Could you check a few things on this model? Use its own coordinates, in mm. A direction names the side the tool comes from. Coordinates: 2 decimals unless noted, no trailing zeros. Order: outer loops, then holes, each group sorted by start corner. A loop starts at its lowest first (then second) coordinate and runs counter-clockwise, first axis right, second up. Notation, with made-up numbers: M 6,-22.75 L 46,-22.75 A15 ccw 46,-3.75 Z; hole C 59,71.5 d8. An arc over 180 degrees is marked long. Put each result on its own line as item: value. Start each with the question number.
```python
from build123d import *

# Parameters (mm, degrees)
SKETCH_1_W               = 370
SKETCH_1_H               = 370
EXTRUDE_1_DEPTH          = 15
SKETCH_2_W               = 155
SKETCH_2_H               = 155
CUT_EXTRUDE_1_DEPTH      = 20
HOLE_WIZARD_1_AT_2_COUNT = 2
HOLE_WIZARD_1_AT_2_PITCH = 320
HOLE_WIZARD_1_AT_3_COUNT = 2
HOLE_WIZARD_1_AT_3_PITCH = 226.27416998
HOLE_WIZARD_1_AT_4_COUNT = 2
HOLE_WIZARD_1_AT_4_PITCH = 226.27416998
MM_1_D                   = 20
MM_1_DEPTH               = 17
MM_1_CSINK_D             = 20.05
MM_1_CSINK_ANGLE         = 90
MM_1_TIP                 = 6.00860619


with BuildPart() as part:
    # 草图1 → 凸台-拉伸1 (new body)
    with BuildSketch(Plane.XY):
        Rectangle(SKETCH_1_W, SKETCH_1_H)
    extrude(amount=EXTRUDE_1_DEPTH)

    # 草图2 → 切除-拉伸1 (cut)
    with BuildSketch(Plane.XY.offset(15)):
        with Locations((107.5, 107.5)):
            Rectangle(SKETCH_2_W, SKETCH_2_H)
        with Locations((-107.5, 107.5)):
            Rectangle(SKETCH_2_W, SKETCH_2_H)
        with Locations((-107.5, -107.5)):
            Rectangle(SKETCH_2_W, SKETCH_2_H)
        with Locations((107.5, -107.5)):
            Rectangle(SKETCH_2_W, SKETCH_2_H)
    extrude(amount=-CUT_EXTRUDE_1_DEPTH, mode=Mode.SUBTRACT)

    # 草图4 → 打孔尺寸(%根据)内六角圆柱头螺钉的类型1 (revolve, cut)
    with BuildSketch(Plane(origin=(-160, 0, 15), x_dir=(0, -1, 0), z_dir=(1, 0, 0))):
        Polygon((0, 0), (0, 20.304733405), (5.5, 17), (5.5, 11), (9, 11), (9, 0.025), (9.025, 0), align=None)
    hole_wizard_1 = revolve(axis=Axis((-160, 0, 21.35), (0, 0, -1)), mode=Mode.SUBTRACT)

    # 打孔尺寸(%根据)内六角圆柱头螺钉的类型1 at 2: 打孔尺寸(%根据)内六角圆柱头螺钉的类型1 ×2
    with Locations(*[(i * HOLE_WIZARD_1_AT_2_PITCH, 0, 0) for i in range(1, HOLE_WIZARD_1_AT_2_COUNT)]):
        add(hole_wizard_1, mode=Mode.SUBTRACT)

    # 打孔尺寸(%根据)内六角圆柱头螺钉的类型1 at 3: 打孔尺寸(%根据)内六角圆柱头螺钉的类型1 ×2
    with Locations(*[Vector(0.707106781, 0.707106781, 0) * (i * HOLE_WIZARD_1_AT_3_PITCH) for i in range(1, HOLE_WIZARD_1_AT_3_COUNT)]):
        add(hole_wizard_1, mode=Mode.SUBTRACT)

    # 打孔尺寸(%根据)内六角圆柱头螺钉的类型1 at 4: 打孔尺寸(%根据)内六角圆柱头螺钉的类型1 ×2
    with Locations(*[Vector(0.707106781, -0.707106781, 0) * (i * HOLE_WIZARD_1_AT_4_PITCH) for i in range(1, HOLE_WIZARD_1_AT_4_COUNT)]):
        add(hole_wizard_1, mode=Mode.SUBTRACT)

    # 大小mm 暗销槽口1
    with Locations(Plane.XY.offset(15)):
        with Locations((0, 0)):
            CounterSinkHole(MM_1_D / 2, MM_1_CSINK_D / 2, depth=MM_1_DEPTH, counter_sink_angle=MM_1_CSINK_ANGLE)
            with Locations((0, 0, -(MM_1_DEPTH + MM_1_TIP / 2))):  # 118° drill point
                Cone(0, MM_1_D / 2, MM_1_TIP, mode=Mode.SUBTRACT)


solid = part.part
```
Item 1: I need wall thicknesses on probe 1 along X at (y, z) = (0, 3.15); probe 2 along X at (y, z) = (0, 9). Which ranges of each line are inside material? Lowest first, please.
Item 2: For pin 1 Ø20 at (x, y) = (1.5, -163) entering from +Z; pin 2 Ø4.5 at (y, z) = (-101.5, 9) entering from -X; pin 3 Ø7.5 at (x, z) = (77.5, 4.5) entering from +Y; pin 4 Ø4.5 at (x, z) = (-74, 7.5) entering from -Y, each with a flat end and sliding along its axis, tell me the tip position at first contact or that it passes through.
Item 3: If we mould it in two halves opening along Y, with no side actions, what happens to faces 4 (the flat face through (0, 185, 7)), 5 (the flat face through (-185, 0, 7)), 6 (the cylindrical face through (-154.63, 1.19, 2.03))? For each: released by +Y, released by -Y, zero draft, split by the parting line, or undercut.
Item 4: If we section it at C-C on x = -160: Write out the boundary of the cut face in (y, z) (3 decimals).
Item 5: For faces 1 (the flat face through (30, 106, 8)), 2 (the flat face through (-164, 4, 4)), 3 (the flat face through (-30, -109, 8)), which set-ups out of +Z, -Z, +X, -X, +Y, -Y let a thin tool reach every point of the face, with its end or its side?
Item 6: If we section it at B-B on y = 0: State how many separate pieces and enclosed holes the cut face has, then the cut area to 3 significant figures.
Item 7: If we section it at A-A on z = 9.75: Write out the boundary of the cut face in (x, y), then the cut area to 3 significant figures.
Geometry check:
1. probe 1: x = -185 to -165.5, -154.5 to -10, 10 to 154.5, 165.5 to 185
1. probe 2: x = -185 to -169, -151 to -10, 10 to 151, 169 to 185
2. pin 1: stops at z = 15
2. pin 2: stops at x = -30
2. pin 3: stops at y = 30
2. pin 4: stops at y = -30
3. face 4: released by +Y
3. face 5: zero draft
3. face 6: undercut
4. outline: M -30,0 L -5.5,0 L -5.5,4 L -9,4 L -9,14.975 L -9.025,15 L -30,15 Z; M 5.5,0 L 30,0 L 30,15 L 9.025,15 L 9,14.975 L 9,4 L 5.5,4 Z
5. face 1: +Z, -Z, +X, +Y
5. face 2: +Z
5. face 3: +Z, -Z, -X, -Y
6. separate pieces: 4
6. enclosed holes: 0
6. area: 4,770 mm²
7. outline: M -185,-30 L -30,-30 L -30,-185 L 30,-185 L 30,-30 L 185,-30 L 185,30 L 30,30 L 30,185 L -30,185 L -30,30 L -185,30 Z; hole C -160,0 d18; hole C 0,0 d20; hole C 0,-160 d18; hole C 0,160 d18; hole C 160,0 d18
7. area: 39,500 mm²
